Verification items for the finished model (mm, model axes). A direction names the side the tool comes from. Give positions to 0.01 mm unless a question says otherwise; leave off trailing zeros. Write each loop counter-clockwise with the first axis right and the second up, starting at its lowest first coordinate (ties: lowest second). Pieces come first, ordered by that corner, then holes. Notation, with made-up numbers: (18.25, -18.75) - (44.25, -18.75) arc R9 cw to (44.25, -8.75) - close; hole circle Ø6 at (22, 58.25). An arc over 180 degrees is marked (long way). Put each result on its own line as item: value.
from build123d import *

# Parameters (mm, degrees)
SKETCH_1_W               = 20.5
SKETCH_1_H               = 15
EXTRUDE_1_DEPTH          = 15
CUT_EXTRUDE_1_DEPTH      = 27.485845276
CUT_EXTRUDE_1_DEPTH_BACK = 7.5
SKETCH_2_R               = 5
SKETCH_4_W               = 5.6
SKETCH_4_H               = 4.7
CUT_EXTRUDE_4_DEPTH      = 10
SKETCH_5_W               = 9.5
SKETCH_5_H               = 7
CUT_EXTRUDE_5_DEPTH      = 20.654834011
CUT_EXTRUDE_2_DEPTH      = 7.3
CUT_EXTRUDE_6_DEPTH      = 24.55976443
CUT_EXTRUDE_START        = -1.8
CUT_EXTRUDE_7_DEPTH      = 10.6
SKETCH_11_W              = 15.106844648
SKETCH_11_H              = 10.6
CUT_EXTRUDE_8_DEPTH      = 2
SKETCH_12_R              = 7.5
CUT_EXTRUDE_9_DEPTH      = 7
CHAMFER_1_SIZE           = 0.4
CHAMFER_2_SIZE           = 0.4
CHAMFER_4_SIZE           = 0.8
CHAMFER_7_SIZE           = 0.8
CHAMFER_8_SIZE           = 0.4


# Some blends are built 0.0001 mm under size
with BuildPart() as part:
    # 草图1 → 凸台-拉伸1 (new body)
    with BuildSketch(Plane.XY):
        Rectangle(SKETCH_1_W, SKETCH_1_H)
    extrude(amount=EXTRUDE_1_DEPTH)

    # 草图2 → 切除-拉伸1 (cut, two sides: drawn at the far end of the back side and taken through both)
    with BuildSketch(Plane(origin=(10.25, 0, 0), x_dir=(0, 0, -1), z_dir=(1, 0, 0)).offset(-CUT_EXTRUDE_1_DEPTH_BACK)):
        with Locations((-17.541169992, 0)):
            Circle(SKETCH_2_R)
        with Locations((3.030989937, 0)):
            Circle(SKETCH_2_R)
    extrude(amount=CUT_EXTRUDE_1_DEPTH + CUT_EXTRUDE_1_DEPTH_BACK, mode=Mode.SUBTRACT)

    # 草图4 → 切除-拉伸4 (cut)
    with BuildSketch(Plane.XY.offset(15)):
        with Locations((5.75, 0)):
            Rectangle(SKETCH_4_W, SKETCH_4_H)
    extrude(amount=-CUT_EXTRUDE_4_DEPTH, mode=Mode.SUBTRACT)

    # 草图5 → 切除-拉伸5 (cut, through all)
    with BuildSketch(Plane.XY.offset(15)):
        with Locations((-5.5, 0)):
            Rectangle(SKETCH_5_W, SKETCH_5_H)
    extrude(amount=-CUT_EXTRUDE_5_DEPTH, mode=Mode.SUBTRACT)

    # 草图3 → 切除-拉伸2 (cut)
    with BuildSketch(Plane(origin=(10.25, 0, 0), x_dir=(0, 0, -1), z_dir=(1, 0, 0))):
        with BuildLine():
            Line((-9.612291748, -0.57471402), (-8.843502884, -1.343502884))
            ThreePointArc((-8.843502884, -1.343502884), (-5.6, 0), (-8.843502884, 1.343502884))
            Line((-8.843502884, 1.343502884), (-9.612291748, 0.57471402))
            Line((-9.612291748, 0.57471402), (-9.612291748, -0.57471402))
        make_face()
    extrude(amount=-CUT_EXTRUDE_2_DEPTH, mode=Mode.SUBTRACT)

    # 草图9 → 切除-拉伸6 (cut, through all)
    with BuildSketch(Plane(origin=(0, 7.5, 0), x_dir=(1, 0, 0), z_dir=(0, 1, 0))):
        with BuildLine():
            Line((-7.8, -7.25), (-7.8, -7.75))
            ThreePointArc((-7.8, -7.75), (-7.605892808, -8.725842753), (-7.053122292, -9.553122292))
            Line((-7.053122292, -9.553122292), (-6.188762276, -10.417482308))
            Line((-6.188762276, -10.417482308), (-4.311237724, -10.417482308))
            Line((-4.311237724, -10.417482308), (-3.446877708, -9.553122292))
            ThreePointArc((-3.446877708, -9.553122292), (-2.894107192, -8.725842753), (-2.7, -7.75))
            Line((-2.7, -7.75), (-2.7, -7.25))
            ThreePointArc((-2.7, -7.25), (-5.25, -4.7), (-7.8, -7.25))
        make_face()
    extrude(amount=-CUT_EXTRUDE_6_DEPTH, mode=Mode.SUBTRACT)

    # 草图10 → 切除-拉伸7 (cut)
    with BuildSketch(Plane.XZ.offset(-3.5).offset(CUT_EXTRUDE_START)):
        with BuildLine():
            Line((-5.25, 13.5), (-10.25, 13.5))
            Line((-10.25, 13.5), (-10.25, 1.5))
            Line((-10.25, 1.5), (-5.25, 1.5))
            ThreePointArc((-5.25, 1.5), (0.75, 7.5), (-5.25, 13.5))
        make_face()
    extrude(amount=CUT_EXTRUDE_7_DEPTH, mode=Mode.SUBTRACT)

    # 草图11 → 切除-拉伸8 (cut)
    with BuildSketch(Plane.ZY.offset(10.25)):
        with Locations((7.446577676, 0)):
            Rectangle(SKETCH_11_W, SKETCH_11_H)
    extrude(amount=-CUT_EXTRUDE_8_DEPTH, mode=Mode.SUBTRACT)

    # 草图12 → 切除-拉伸9 (cut)
    with BuildSketch(Plane.XZ.offset(-3.5)):
        with Locations((-5.25, 7.5)):
            Circle(SKETCH_12_R)
    extrude(amount=CUT_EXTRUDE_9_DEPTH, mode=Mode.SUBTRACT)

    # 倒角1
    chamfer_1_edges = [part.edges().sort_by_distance(p)[0] for p in [
        (10.25, 5.903047554, 15),
        (10.25, -5.738284436, 0),
        (10.25, -5.903047554, 15),
        (10.25, 0, 12.541169992),
        (10.25, 0, 1.969010063),
        (10.25, 5.738284436, 0),
        (10.25, 7.5, 7.5),
        (10.25, -7.5, 7.5),
    ]]
    chamfer(chamfer_1_edges, length=CHAMFER_1_SIZE)

    # 倒角2
    chamfer_2_edges = [part.edges().sort_by_distance(p)[0] for p in [
        (-0.2, 7.5, 15),
        (-0.2, 7.5, 0),
        (-0.2, -7.5, 0),
        (-10.25, 7.5, 7.5),
        (-10.25, -7.5, 7.5),
        (-0.2, -7.5, 15),
    ]]
    chamfer(chamfer_2_edges, length=CHAMFER_2_SIZE)

    # 倒角4
    chamfer_4_edges = [part.edges().sort_by_distance(p)[0] for p in [
        (-10.25, 6.2, 0),
        (-10.25, -6.2, 0),
        (-10.25, -6.2, 15),
        (-10.25, 6.2, 15),
    ]]
    chamfer(chamfer_4_edges, length=CHAMFER_4_SIZE - 0.0001)  # a hair under: the kernel refuses the full size

    # 倒角7
    # the kernel refuses this chamfer: 0.8 mm, written as the material it takes off along each edge
    with BuildSketch(Plane(origin=(2.95, -2.35, 13.127837918), x_dir=(0, -0.8336429325250914, 0.5523037760607525), z_dir=(1, 0, 0))) as chamfer_7_piece_1:
        with BuildLine():
            Line((0.956878157, 0), (-CHAMFER_7_SIZE * 0.552303776061, CHAMFER_7_SIZE * 0.833642932525))
            Line((-CHAMFER_7_SIZE * 0.552303776061, CHAMFER_7_SIZE * 0.833642932525), (0, 0))
            ThreePointArc((0, 0), (0.492968028, 0.022921924), (0.956878157, 0))
        make_face()
    extrude(amount=5.6, mode=Mode.SUBTRACT)
    with BuildSketch(Plane(origin=(2.95, 2.35, 13.127837918), x_dir=(0, 0.8336429325250913, 0.5523037760607528), z_dir=(1, 0, 0))) as chamfer_7_piece_2:
        with BuildLine():
            Line((0.956878157, 0), (-CHAMFER_7_SIZE * 0.552303776061, -CHAMFER_7_SIZE * 0.833642932525))
            Line((-CHAMFER_7_SIZE * 0.552303776061, -CHAMFER_7_SIZE * 0.833642932525), (0, 0))
            ThreePointArc((0, 0), (0.492968028, -0.022921924), (0.956878157, 0))
        make_face()
    extrude(amount=5.6, mode=Mode.SUBTRACT)

    # 倒角8
    chamfer_8_edges = [part.edges().sort_by_distance(p)[0] for p in [
        (2.75, 0, 0),
        (-4.5, -3.5, 0),
        (-0.75, 0, 0),
        (-4.5, 3.5, 0),
    ]]
    chamfer(chamfer_8_edges, length=CHAMFER_8_SIZE)


solid = part.part
Q1. Scan lines: line 1 along X through (y, z) = (-1, 12); line 2 along Y through (x, z) = (9, 7.5); line 3 along Z through (x, y) = (-5, -4.75). Record each from-to range of solid material in increasing order.
Answers follow:
line 1: x = 0.75 to 2.95, 8.55 to 10.25
line 2: y = -7.5 to -1.9, 1.9 to 7.5
line 3: z = 0 to 1.51, 13.49 to 15
Q2. Section check A-A, the plane z = 7.5. Give the number of separate pieces and of enclosed holes in the cut face, plus the area to 3 significant figures.
Answers follow:
separate pieces: 3
enclosed holes: 0
area: 125 mm2
Q3. Section check D-D, the plane z = 2.75. Record the cut outline in (x, y), plus the area to 3 significant figures.
Answers follow:
outline: (-10.25, -7.1) - (-9.85, -7.5) - (9.85, -7.5) - (10.25, -7.1) - (10.25, 7.1) - (9.85, 7.5) - (-9.85, 7.5) - (-10.25, 7.1) - (-10.25, 5.3) - (-1.58, 5.3) - (-1.58, 3.5) - (0.55, 3.5) - (0.55, -3.5) - (-1.58, -3.5) - (-1.58, -5.3) - (-10.25, -5.3) - close
area: 200 mm2
Q4. Set-up check for faces 1 (the face through (6, 0, 5)), 2 (the face through (-7, 4, 1.5)), 3 (the face through (-5, -6, 10.417)): record each of +Z, -Z, +X, -X, +Y, -Y from which the full face is reachable in a straight line by a thin tool's end or side.
Answers follow:
face 1: +Z
face 2: -X
face 3: +Y, -Y
Q5. Release check for a two-part mould opening along X. For faces 4 (the face through (9.41, -0.06, 5.6)), 5 (the face through (0.75, -4.39, 7.37)), 6 (the face through (6, -2.35, 9)), 7 (the face through (-5.2, 6.4, 4.7)) record: released by +X, released by -X, zero draft, split by the parting line, or undercut.
Answers follow:
face 4: zero draft
face 5: released by -X
face 6: undercut
face 7: undercut
Q6. Section check B-B, the plane y = 0. Record the cut outline in (x, z).
Answers follow:
outline: (-0.75, 0.4) - (-0.35, 0) - (2.35, 0) - (2.75, 0.4) - (2.75, 1.97) - (9.85, 1.97) - (10.25, 2.37) - (10.25, 5.6) - (8.55, 5.6) - (8.55, 5) - (2.95, 5) - (2.95, 12.54) - (2.75, 12.54) - (2.75, 15) - (-0.75, 15) - (-0.75, 13.5) arc R7.5 cw to (-0.75, 1.5) - close; (8.55, 9.61) - (10.25, 9.61) - (10.25, 12.14) - (9.85, 12.54) - (8.55, 12.54) - close
Q7. Go/stop test with flat-tipped pins: pin 1 Ø4 at (x, y) = (5.5, 0) entering from +Z; pin 2 Ø1.2 at (y, z) = (4.5, 1) entering from -X; pin 3 Ø2 at (y, z) = (3, 10) entering from -X. Record where each tip stops, or that it passes through.
Answers follow:
pin 1: stops at z = 5
pin 2: stops at x = -8.25
pin 3: stops at x = -0.28
Q8. Section check C-C, the plane x = 9.25. Record the cut outline in (y, z).
Answers follow:
outline: (-7.5, 0.4) - (-7.1, 0) - (-3.98, 0) arc R5 cw to (3.98, 0) - (7.1, 0) - (7.5, 0.4) - (7.5, 14.6) - (7.1, 15) - (4.31, 15) arc R5 cw to (-4.31, 15) - (-7.1, 15) - (-7.5, 14.6) - close; hole (-1.34, 8.84) arc R1.9 ccw (long way) to (1.34, 8.84) - (0.57, 9.61) - (-0.57, 9.61) - close
